from build123d import *

# Parameters (mm, degrees)
SKETCH1_R               = 2.6035
BOSS_EXTRUDE1_DEPTH     = 457.2
CUT_EXTRUDE2_DEPTH      = 4.318
CUT_EXTRUDE2_DEPTH_BACK = 26.924
SKETCH4_W               = 10.066529056
SKETCH4_H               = 26.230878965
CUT_EXTRUDE3_DEPTH      = 26.4


with BuildPart() as part:
    # Sketch1 → Boss-Extrude1 (new body, symmetric)
    with BuildSketch(Plane.XY):
        with BuildLine():
            Line((-7.179650497, -8.645192506), (-3.952270251, -5.423690499))
            ThreePointArc((-3.952270251, -5.423690499), (-2.922936451, -4.736929036), (-1.709253557, -4.4958))
            Line((-1.709253557, -4.4958), (1.709253557, -4.4958))
            ThreePointArc((1.709253557, -4.4958), (2.922936451, -4.736929036), (3.952270251, -5.423690499))
            Line((3.952270251, -5.423690499), (7.179650497, -8.645192506))
            ThreePointArc((7.179650497, -8.645192506), (7.41473083, -9.822813117), (6.416408329, -10.4902))
            Line((6.416408329, -10.4902), (4.287512407, -10.4902))
            ThreePointArc((4.287512407, -10.4902), (3.54574862, -10.79744862), (3.2385, -11.539212407))
            Line((3.2385, -11.539212407), (3.2385, -11.650987593))
            ThreePointArc((3.2385, -11.650987593), (3.54574862, -12.39275138), (4.287512407, -12.7))
            Line((4.287512407, -12.7), (5.317126718, -12.7))
            ThreePointArc((5.317126718, -12.7), (5.825126718, -12.192), (6.333126718, -12.7))
            Line((6.333126718, -12.7), (9.550443118, -12.7))
            ThreePointArc((9.550443118, -12.7), (10.058366869, -12.192000006), (10.566443095, -12.699847501))
            ThreePointArc((10.566443095, -12.699847501), (12.082537762, -12.08250727), (12.699846982, -10.566399977))
            ThreePointArc((12.699846982, -10.566399977), (12.192000006, -10.058323491), (12.7, -9.5504))
            Line((12.7, -9.5504), (12.7, -6.3330836))
            ThreePointArc((12.7, -6.3330836), (12.192, -5.8250836), (12.7, -5.3170836))
            Line((12.7, -5.3170836), (12.7, -4.287469289))
            ThreePointArc((12.7, -4.287469289), (12.39275138, -3.545705502), (11.650987593, -3.238456882))
            Line((11.650987593, -3.238456882), (11.539212407, -3.238456882))
            ThreePointArc((11.539212407, -3.238456882), (10.79744862, -3.545705502), (10.4902, -4.287469289))
            Line((10.4902, -4.287469289), (10.4902, -6.402089023))
            ThreePointArc((10.4902, -6.402089023), (9.856505071, -7.351067942), (8.737131347, -7.129408934))
            Line((8.737131347, -7.129408934), (5.441005833, -3.840816462))
            ThreePointArc((5.441005833, -3.840816462), (4.750877967, -2.809883091), (4.5085, -1.593185507))
            Line((4.5085, -1.593185507), (4.5085, 1.593185507))
            ThreePointArc((4.5085, 1.593185507), (4.750877967, 2.809883091), (5.441005833, 3.840816462))
            Line((5.441005833, 3.840816462), (8.737131347, 7.129408934))
            ThreePointArc((8.737131347, 7.129408934), (9.856505071, 7.351067942), (10.4902, 6.402089023))
            Line((10.4902, 6.402089023), (10.4902, 4.287469289))
            ThreePointArc((10.4902, 4.287469289), (10.79744862, 3.545705502), (11.539212407, 3.238456882))
            Line((11.539212407, 3.238456882), (11.650987593, 3.238456882))
            ThreePointArc((11.650987593, 3.238456882), (12.39275138, 3.545705502), (12.7, 4.287469289))
            Line((12.7, 4.287469289), (12.7, 5.3170836))
            ThreePointArc((12.7, 5.3170836), (12.192, 5.8250836), (12.7, 6.3330836))
            Line((12.7, 6.3330836), (12.7, 9.5504))
            ThreePointArc((12.7, 9.5504), (12.192000006, 10.058323491), (12.699846982, 10.566399977))
            ThreePointArc((12.699846982, 10.566399977), (12.082537762, 12.08250727), (10.566443095, 12.699847501))
            ThreePointArc((10.566443095, 12.699847501), (10.058366869, 12.192000006), (9.550443118, 12.7))
            Line((9.550443118, 12.7), (6.333126718, 12.7))
            ThreePointArc((6.333126718, 12.7), (5.825126718, 12.192), (5.317126718, 12.7))
            Line((5.317126718, 12.7), (4.287512407, 12.7))
            ThreePointArc((4.287512407, 12.7), (3.54574862, 12.39275138), (3.2385, 11.650987593))
            Line((3.2385, 11.650987593), (3.2385, 11.539212407))
            ThreePointArc((3.2385, 11.539212407), (3.54574862, 10.79744862), (4.287512407, 10.4902))
            Line((4.287512407, 10.4902), (6.476788598, 10.4902))
            ThreePointArc((6.476788598, 10.4902), (7.432222385, 9.85140422), (7.207036008, 8.724370562))
            Line((7.207036008, 8.724370562), (3.898272566, 5.423169045))
            ThreePointArc((3.898272566, 5.423169045), (2.869120213, 4.736787962), (1.655778399, 4.4958))
            Line((1.655778399, 4.4958), (-1.655778399, 4.4958))
            ThreePointArc((-1.655778399, 4.4958), (-2.869120213, 4.736787962), (-3.898272566, 5.423169045))
            Line((-3.898272566, 5.423169045), (-7.207036008, 8.724370562))
            ThreePointArc((-7.207036008, 8.724370562), (-7.432222385, 9.85140422), (-6.476788598, 10.4902))
            Line((-6.476788598, 10.4902), (-4.287512407, 10.4902))
            ThreePointArc((-4.287512407, 10.4902), (-3.54574862, 10.79744862), (-3.2385, 11.539212407))
            Line((-3.2385, 11.539212407), (-3.2385, 11.650987593))
            ThreePointArc((-3.2385, 11.650987593), (-3.54574862, 12.39275138), (-4.287512407, 12.7))
            Line((-4.287512407, 12.7), (-5.317126718, 12.7))
            ThreePointArc((-5.317126718, 12.7), (-5.825126718, 12.192), (-6.333126718, 12.7))
            Line((-6.333126718, 12.7), (-9.550443118, 12.7))
            ThreePointArc((-9.550443118, 12.7), (-10.058366869, 12.192000006), (-10.566443095, 12.699847501))
            ThreePointArc((-10.566443095, 12.699847501), (-12.082537762, 12.08250727), (-12.699846982, 10.566399977))
            ThreePointArc((-12.699846982, 10.566399977), (-12.192000006, 10.058323491), (-12.7, 9.5504))
            Line((-12.7, 9.5504), (-12.7, 6.3330836))
            ThreePointArc((-12.7, 6.3330836), (-12.192, 5.8250836), (-12.7, 5.3170836))
            Line((-12.7, 5.3170836), (-12.7, 4.287469289))
            ThreePointArc((-12.7, 4.287469289), (-12.39275138, 3.545705502), (-11.650987593, 3.238456882))
            Line((-11.650987593, 3.238456882), (-11.539212407, 3.238456882))
            ThreePointArc((-11.539212407, 3.238456882), (-10.79744862, 3.545705502), (-10.4902, 4.287469289))
            Line((-10.4902, 4.287469289), (-10.4902, 6.402089023))
            ThreePointArc((-10.4902, 6.402089023), (-9.856505071, 7.351067942), (-8.737131347, 7.129408934))
            Line((-8.737131347, 7.129408934), (-5.441005833, 3.840816462))
            ThreePointArc((-5.441005833, 3.840816462), (-4.750877967, 2.809883091), (-4.5085, 1.593185507))
            Line((-4.5085, 1.593185507), (-4.5085, -1.593185507))
            ThreePointArc((-4.5085, -1.593185507), (-4.750877967, -2.809883091), (-5.441005833, -3.840816462))
            Line((-5.441005833, -3.840816462), (-8.737131347, -7.129408934))
            ThreePointArc((-8.737131347, -7.129408934), (-9.856505071, -7.351067942), (-10.4902, -6.402089023))
            Line((-10.4902, -6.402089023), (-10.4902, -4.287469289))
            ThreePointArc((-10.4902, -4.287469289), (-10.79744862, -3.545705502), (-11.539212407, -3.238456882))
            Line((-11.539212407, -3.238456882), (-11.650987593, -3.238456882))
            ThreePointArc((-11.650987593, -3.238456882), (-12.39275138, -3.545705502), (-12.7, -4.287469289))
            Line((-12.7, -4.287469289), (-12.7, -5.3170836))
            ThreePointArc((-12.7, -5.3170836), (-12.192, -5.8250836), (-12.7, -6.3330836))
            Line((-12.7, -6.3330836), (-12.7, -9.5504))
            ThreePointArc((-12.7, -9.5504), (-12.192000006, -10.058323491), (-12.699846982, -10.566399977))
            ThreePointArc((-12.699846982, -10.566399977), (-12.082537762, -12.08250727), (-10.566443095, -12.699847501))
            ThreePointArc((-10.566443095, -12.699847501), (-10.058366869, -12.192000006), (-9.550443118, -12.7))
            Line((-9.550443118, -12.7), (-6.333126718, -12.7))
            ThreePointArc((-6.333126718, -12.7), (-5.825126718, -12.192), (-5.317126718, -12.7))
            Line((-5.317126718, -12.7), (-4.287512407, -12.7))
            ThreePointArc((-4.287512407, -12.7), (-3.54574862, -12.39275138), (-3.2385, -11.650987593))
            Line((-3.2385, -11.650987593), (-3.2385, -11.539212407))
            ThreePointArc((-3.2385, -11.539212407), (-3.54574862, -10.79744862), (-4.287512407, -10.4902))
            Line((-4.287512407, -10.4902), (-6.416408329, -10.4902))
            ThreePointArc((-6.416408329, -10.4902), (-7.41473083, -9.822813117), (-7.179650497, -8.645192506))
        make_face()
        Circle(SKETCH1_R, mode=Mode.SUBTRACT)
    extrude(amount=BOSS_EXTRUDE1_DEPTH, both=True)

    # Sketch3 → Cut-Extrude2 (cut, two sides)
    with BuildSketch(Plane.ZY.offset(12.7)) as cut_extrude2_sk:
        Polygon((-203.2, -27.552777595), (-203.2, 21.158109763), (-461.090893327, 21.158109763), (-461.090893327, -25.4), align=None)
    extrude(amount=CUT_EXTRUDE2_DEPTH, mode=Mode.SUBTRACT)
    extrude(cut_extrude2_sk.sketch, amount=-CUT_EXTRUDE2_DEPTH_BACK, mode=Mode.SUBTRACT)

    # Sketch4 → Cut-Extrude3 (cut, through all)
    with BuildSketch(Plane(origin=(12.7, 0, 0), x_dir=(0, 0, -1), z_dir=(1, 0, 0))):
        Polygon((144.651128895, 14.668633048), (144.651128895, -33.454509464), (-421.914129737, -33.454509464), (-459.790894846, -33.454509464), (-459.790894846, 14.668633048), (-421.914129737, 14.668633048), align=None)
        with Locations((199.285393072, 0.039458439)):
            Rectangle(SKETCH4_W, SKETCH4_H)
    extrude(amount=-CUT_EXTRUDE3_DEPTH, mode=Mode.SUBTRACT)


solid = part.part
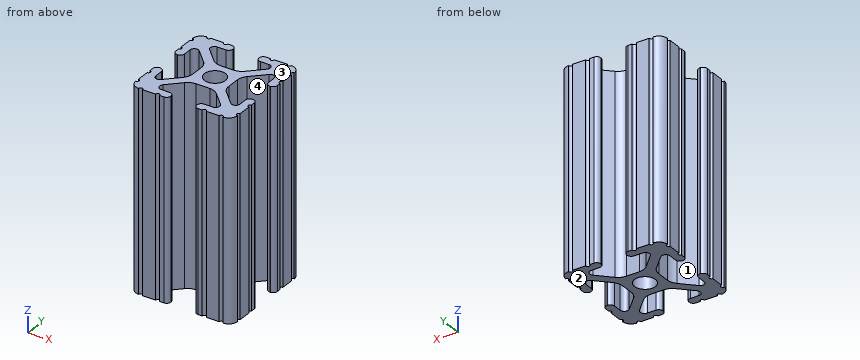
Verification items for the finished model (mm, model axes). Face numbers are marked on the shaded views. A direction names the side the tool comes from. Give positions to 0.01 mm unless a question says otherwise; leave off trailing zeros. Loops run counter-clockwise (first coordinate to the right, second up) from the corner with the lowest first, then second, coordinate; pieces in that order, holes last. Notation, with made-up numbers: (16, 62.25) - (30, 62.25) arc R20 cw to (30, 96.25) - close; hole circle Ø2 at (76.5, -24). An arc over 180 degrees is marked (long way). Write each question's results on one line, items separated by ' | '.
1) Depth check by flat-ended pin: P1, Ø2.5, axis at y = -0.5, z = -172.5, coming from the -X side; P2, Ø3, axis at y = -1, z = -164, coming from the -X side; P3, Ø2, axis at y = -3, z = -180.5, coming from the +X side. Enter the tip coordinate at first touch or a pass-through.
Solution:
P1: x = -4.51 | P2: x = -4.64 | P3: x = 12.66
2) Sectioned sample at B-B on x = 0. Record the boundary of the cut face in (y, z).
Solution:
outline: (-4.5, -194.25) - (-2.6, -194.25) - (-2.6, -144.65) - (-4.5, -144.65) - close; (2.6, -194.25) - (4.5, -194.25) - (4.5, -144.65) - (2.6, -144.65) - close
3) Tool access check on the marked faces 3 and 4. Record the directions out of +Z, -Z, +X, -X, +Y, -Y that give a thin tool (end or side, any length) a straight path to the whole face; none if there is none.
Solution:
face 3: +Z, +X, -X, +Y, -Y | face 4: +Z, -Z
4) Sectioned sample at A-A on y = 0. Record the boundary of the cut face in (x, z), plus the area to 3 significant figures.
Solution:
outline: (-4.51, -194.25) - (-2.6, -194.25) - (-2.6, -144.65) - (-4.51, -144.65) - close; (2.6, -194.25) - (4.51, -194.25) - (4.51, -144.65) - (2.6, -144.65) - close | area: 189 mm2
5) Mould release check, pull along Y, two halves, no side actions. Record for the marked faces 1 and 2: pulls with the +Y half, pulls with the -Y half, needs draft (parallel to the pull), parting line crosses it, or undercut.
Solution:
face 1: undercut | face 2: needs draft
6) Material ranges on L1, parallel to X at y = 0, z = -161; L2, parallel to Y at x = 0, z = -162; L3, parallel to X at y = 7.25, z = -156, recorded low to high. Write a range as from..to.
Solution:
L1: -4.51..-2.6, 2.6..4.51 | L2: -4.5..-2.6, 2.6..4.5 | L3: -12.7..-10.04, -8.88..-5.73, 5.73..8.88, 10.04..12.7
